Can you work these out from the model? Positions are in its coordinate system, mm. Face numbers are marked on the shaded views. A direction names the side the tool comes from. Round coordinates to 2 decimals unless told otherwise and drop trailing zeros. Write each loop counter-clockwise with the first axis right and the second up, starting at its lowest first coordinate (ties: lowest second). Pieces come first, ordered by that corner, then holes. Notation, with made-up numbers: (-21, -25) - (31, -25) arc R18 ccw to (31, -4) - close; hole circle Ø1 at (51.5, -21.5). An arc over 180 degrees is marked (long way). One line per item, written item: value. Start each with the question number.
(1) Thinking about a two-plate mould opening in X: for the marked faces 1, 2 and 3, which applies, +X half, -X half, draft (parallel to the pull), parting line (faces both ways), or undercut?
(2) I want a section at D-D on z = 7.5. List the corners of the cut face in (x, y) for me.
(3) On a 3-axis mill with a long thin cutter (end or side, diameter ignored), from which of +Z, -Z, +X, -X, +Y, -Y can I reach the whole of each face in a straight line? I mean the marked faces 4, 5 and 6. Say none if no direction works.
(4) I want a section at C-C on z = -2.5. List the corners of the cut face in (x, y) for me, plus the area to 3 significant figures.
(5) I want a section at A-A on x = -10.5. List the corners of the cut face in (y, z) for me.
(6) I want a section at B-B on y = -5.5. List the corners of the cut face in (x, z) for me.
(7) If I drill on L1, parallel to X at y = -2.5, z = 1.5; L2, parallel to Y at x = 16.5, z = 4.25; L3, parallel to Y at x = -44, z = -4, over which ranges is the centre line in solid material (lowest first)? Write a range as from..to.
(8) I'm going to push flat-ended pins straight in: pin 1 Ø9 at (x, z) = (-61, -0.5) entering from +Y; pin 2 Ø1 at (y, z) = (-23.5, 12.5) entering from +X; pin 3 Ø1 at (x, y) = (-64.5, -20.5) entering from +Z. Where does each tip first touch, or does it pass through?
from build123d import *

# Parameters (mm, degrees)
SKETCH_1_W           = 50
SKETCH_1_H           = 2
SKETCH_1_W_2         = 40
SKETCH_1_H_2         = 20
EXTRUDE_1_DEPTH      = 5
EXTRUDE_1_DEPTH_BACK = 5
EXTRUDE_2_DEPTH      = 10
EXTRUDE_2_DEPTH_BACK = 20


with BuildPart() as part:
    # Sketch 1 → Extrude 1 (new body, two sides)
    with BuildSketch(Plane.XY) as extrude_1_sk:
        Polygon((-74.170588235, -24.287254902), (-22.170588235, -24.287254902), (21.829411765, -24.287254902), (21.829411765, -0.287254902), (-22.170588235, -0.287254902), (-22.170588235, -18.287254902), (-74.170588235, -18.287254902), (-74.170588235, -22.287254902), align=None)
        with Locations((-47.170588235, -21.287254902)):
            Rectangle(SKETCH_1_W, SKETCH_1_H, mode=Mode.SUBTRACT)
        with Locations((-0.170588235, -12.287254902)):
            Rectangle(SKETCH_1_W_2, SKETCH_1_H_2, mode=Mode.SUBTRACT)
    extrude(amount=EXTRUDE_1_DEPTH)
    extrude(extrude_1_sk.sketch, amount=-EXTRUDE_1_DEPTH_BACK)

    # Sketch 2 → Extrude 2 (add, two sides)
    with BuildSketch(Plane.XY.offset(5)) as extrude_2_sk:
        Polygon((-74.170588235, -24.287254902), (-32.170588235, -24.287254902), (-32.170588235, -22.287254902), (-72.170588235, -22.287254902), (-74.170588235, -22.287254902), align=None)
    extrude(amount=EXTRUDE_2_DEPTH)
    extrude(extrude_2_sk.sketch, amount=-EXTRUDE_2_DEPTH_BACK)


solid = part.part
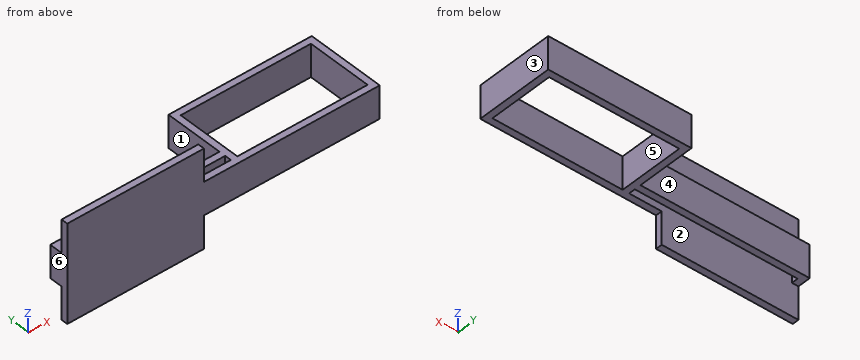
Established:
1. face 1: -X half
1. face 2: undercut
1. face 3: +X half
2. outline: (-74.17, -24.29) - (-32.17, -24.29) - (-32.17, -22.29) - (-74.17, -22.29) - close
3. face 4: +Z, -Z, -X, +Y
3. face 5: +Z, -Z
3. face 6: +Z, -Z, -X, +Y, -Y
4. outline: (-74.17, -24.29) - (21.83, -24.29) - (21.83, -0.29) - (-22.17, -0.29) - (-22.17, -18.29) - (-74.17, -18.29) - close; hole (-72.17, -22.29) - (-22.17, -22.29) - (-22.17, -20.29) - (-72.17, -20.29) - close; hole (-20.17, -22.29) - (19.83, -22.29) - (19.83, -2.29) - (-20.17, -2.29) - close
4. area: 468 mm2
5. outline: (-24.29, -5) - (-22.29, -5) - (-22.29, 5) - (-24.29, 5) - close; (-2.29, -5) - (-0.29, -5) - (-0.29, 5) - (-2.29, 5) - close
6. outline: (-22.17, -5) - (-20.17, -5) - (-20.17, 5) - (-22.17, 5) - close; (19.83, -5) - (21.83, -5) - (21.83, 5) - (19.83, 5) - close
7. L1: -22.17..-20.17, 19.83..21.83
7. L2: -24.29..-22.29, -2.29..-0.29
7. L3: -24.29..-22.29, -20.29..-18.29
8. pin 1: y = -18.29
8. pin 2: x = -32.17
8. pin 3: z = 5
